```python
from build123d import *

# Parameters (mm, degrees)
SKETCH1_R           = 70
BOSS_EXTRUDE1_DEPTH = 50
SKETCH2_R           = 15
BOSS_EXTRUDE2_DEPTH = 50
CUT_EXTRUDE1_DEPTH  = 5


with BuildPart() as part:
    # Sketch1 → Boss-Extrude1 (new body)
    with BuildSketch(Plane(origin=(0, 0, 0), x_dir=(1, 0, 0), z_dir=(0, 1, 0))):
        with Locations(Location((0, 0, 0), (0, 0, 270))):
            Circle(SKETCH1_R)
    extrude(amount=BOSS_EXTRUDE1_DEPTH)

    # Sketch2 → Boss-Extrude2 (add)
    with BuildSketch(Plane(origin=(0, 50, 0), x_dir=(1, 0, 0), z_dir=(0, 1, 0))):
        with Locations(Location((0, 0, 0), (0, 0, 270))):
            Circle(SKETCH2_R)
    extrude(amount=BOSS_EXTRUDE2_DEPTH)

    # Sketch3 → Cut-Extrude1 (cut)
    with BuildSketch(Plane.XZ):
        Polygon((-16.192060877, 11.114878754), (27.540819943, 58.8770179), (10.111567195, 18.864926724), (21.881207876, 18.864926724), (0, -11.114878754), (16.192060877, -11.114878754), (-27.540819943, -58.8770179), (-8.388481815, -16.504098893), (-20.158122496, -16.504098893), (0, 11.114878754), align=None)
    extrude(amount=-CUT_EXTRUDE1_DEPTH, mode=Mode.SUBTRACT)


solid = part.part
```
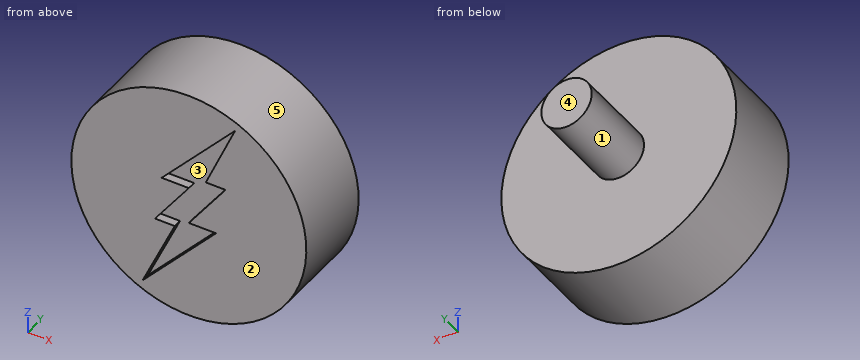
The model under review builds one solid part; all positions refer to its coordinate system, in mm. Face numbers are marked on the shaded views. A direction names the side the tool comes from. Round coordinates to 2 decimals unless told otherwise and drop trailing zeros. Order: outer loops, then holes, each group sorted by start corner. A loop starts at its lowest first (then second) coordinate and runs counter-clockwise, first axis right, second up.
Item 1: Draft analysis for pull direction X (two halves, no side actions). For the marked faces 3, 4 and 5, state which applies: released by +X, released by -X, zero draft, split by the parting line, or undercut.
Working result:
face 3: undercut
face 4: zero draft
face 5: split by the parting line
Item 2: Add section A-A, the plane z = -52.5. State the section outline as (x, y) points, and give its area (3 significant figures).
Working result:
outline: (-46.3, 0) - (-24.66, 0) - (-24.66, 5) - (-21.7, 5) - (-21.7, 0) - (46.3, 0) - (46.3, 50) - (-46.3, 50) - close
area: 4,620 mm2
Item 3: For pin 1 (2.5 mm diameter, centred on x = 18, y = 2.5, fed in from -Z); pin 2 (2.5 mm diameter, centred on x = 9.5, y = 1.5, fed in from -Z); pin 3 (3 mm diameter, centred on x = -15, z = 43, fed in from -Y); pin 4 (3 mm diameter, centred on y = 44, z = -21, fed in from -X), all flat-tipped, find the tip position at first contact; note any pin that passes through.
Working result:
pin 1: stops at z = -67.97
pin 2: stops at z = -69.51
pin 3: stops at y = 0
pin 4: stops at x = -67.23
Item 4: Add section D-D, the plane z = 42.5. State the section outline as (x, y) points, and give its area (3 significant figures).
Working result:
outline: (-55.62, 0) - (12.55, 0) - (12.55, 5) - (20.41, 5) - (20.41, 0) - (55.62, 0) - (55.62, 50) - (-55.62, 50) - close
area: 5,520 mm2
Item 5: Add section C-C, the plane x = 31.5. State the section outline as (y, z) points, and give its area (3 significant figures).
Working result:
outline: (0, -62.51) - (50, -62.51) - (50, 62.51) - (0, 62.51) - close
area: 6,250 mm2
Item 6: To check wall thickness, follow probe 1 along Y at (x, z) = (-63, 3); probe 2 along Z at (x, y) = (-3, 6); probe 3 along Z at (x, y) = (49, 33). State the ranges of each line that lie inside material, in increasing order.
Working result:
probe 1: y = 0 to 50
probe 2: z = -69.94 to 69.94
probe 3: z = -49.99 to 49.99
Item 7: Machinability: for the marked faces 1 and 2, which of the approach directions +Z, -Z, +X, -X, +Y, -Y give a long, thin tool a straight path to every point of the face, cutting with its end or side? Answer none if there is none.
Working result:
face 1: +Y
face 2: +Z, -Z, +X, -X, -Y
Item 8: Add section B-B, the plane y = 16. State the section outline as (x, z) points.
Working result:
outline: circle Ø140 at (0, 0)
